Check sheet for the drawn part. Datum: minimum x, y, z corner. Units: mm. Coordinates: 2 decimals unless noted, no trailing zeros. Order: outer loops, then holes, each group sorted by start corner. A loop starts at its lowest first (then second) coordinate and runs counter-clockwise, first axis right, second up.
1. Cross-section at A-A (x = 101.5). Enter the section's corners in (y, z) (3 decimals), then the cut area to 3 significant figures.
2. Cross-section at B-B (z = 4.75). Enter the section's corners in (x, y) (3 decimals).
3. Gauge pin test, flat ends, axial feed: pin 1 Ø1 at (y, z) = (24.5, 1.5) entering from +X; pin 2 Ø3 at (y, z) = (60, 5) entering from -X; pin 3 Ø1.9 at (y, z) = (3, 4.5) entering from -X. Record the tip position at first contact, or that the pin passes through.
4. Thickness scan on line 1 (Y direction, x = 89, z = 1.5) (3 decimals); line 2 (Y direction, x = 86, z = 3) (3 decimals); line 3 (X direction, y = 65.5, z = 0.5). Record the ranges inside material, lowest first.
5. Cross-section at C-C (y = 75). Enter the section's corners in (x, z), then the cut area to 3 significant figures.
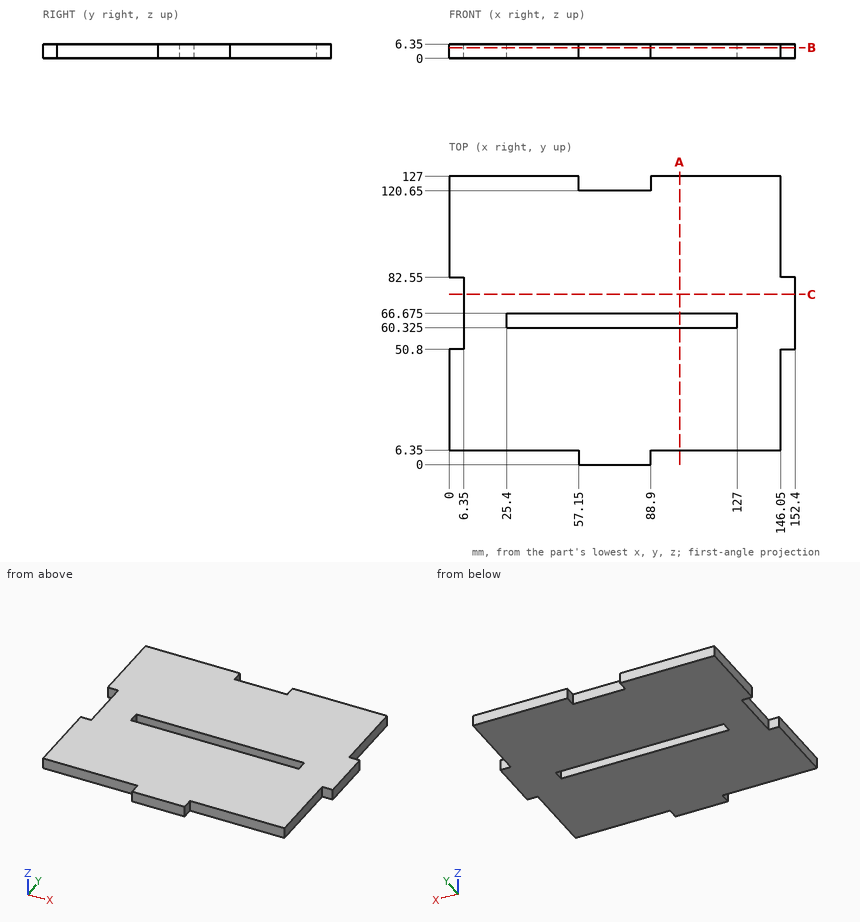
Data:
1. outline: (6.35, 0) - (60.325, 0) - (60.325, 6.35) - (6.35, 6.35) - close; (66.675, 0) - (127, 0) - (127, 6.35) - (66.675, 6.35) - close
1. area: 726 mm2
2. outline: (0, 6.35) - (57.15, 6.35) - (57.15, 0) - (88.9, 0) - (88.9, 6.35) - (146.05, 6.35) - (146.05, 50.8) - (152.4, 50.8) - (152.4, 82.55) - (146.05, 82.55) - (146.05, 127) - (88.9, 127) - (88.9, 120.65) - (57.15, 120.65) - (57.15, 127) - (0, 127) - (0, 82.55) - (6.35, 82.55) - (6.35, 50.8) - (0, 50.8) - close; hole (25.4, 60.325) - (127, 60.325) - (127, 66.675) - (25.4, 66.675) - close
3. pin 1: stops at x = 146.05
3. pin 2: stops at x = 6.35
3. pin 3: stops at x = 57.15
4. line 1: y = 6.35 to 60.325, 66.675 to 127
4. line 2: y = 0 to 60.325, 66.675 to 120.65
4. line 3: x = 6.35 to 25.4, 127 to 152.4
5. outline: (6.35, 0) - (152.4, 0) - (152.4, 6.35) - (6.35, 6.35) - close
5. area: 927 mm2
